Autodesk Inventor part; units mm, degrees
ref_plane "YZ Plane" through (0, 0, 0) normal (1, 0, 0) x (0, 1, 0)
ref_plane "XZ Plane" through (0, 0, 0) normal (0, 1, 0) x (-1, 0, 0)
ref_plane "XY Plane" through (0, 0, 0) normal (0, 0, 1) x (1, 0, 0)
sketch "Sketch2" plane through (0, 0, 0) normal (0, 1, 0) x (-1, 0, 0)
  line L0 (-4, 4) -> (4, 4) construction
  line L1 (4, 4) -> (4, -4) construction
  line L2 (4, -4) -> (-4, -4) construction
  line L3 (-4, -4) -> (-4, 4) construction
  circle A0 centre (0, 0) radius 4
  point P0 (0, 4)
  point P1 (-4, 0)
  dimension "d0" = 8
  dimension "d1" = 8
extrude "Extrusion1" add sketch "Sketch2" along normal blind 3.2
sketch "Sketch10" plane through (0, 0, 0) normal (0, -1, 0) x (1, 0, 0)
  circle A0 centre (0, 0) radius 4
  circle A1 centre (4, 4) radius 2.4 construction
  line L0 (0, 0) -> (4, 4) construction
  circle A2 centre (0, 0) radius 3.2569
  circle A3 centre (0, 0) radius 2.4
  circle A4 centre (0, 0) radius 3.6
  dimension "d92" = 4.8
  dimension "d93" = 4
  dimension "d94" = 4
  dimension "d95" = 4.8
  dimension "d99" = 0.4
extrude "Extrusion6" cut sketch "Sketch10" against normal blind 1.6 contours A3
extrude "Extrusion7" cut sketch "Sketch10" against normal blind 0.4 contours A0
fillet "Fillet1" radius 0.1 1 edges at (4, 3.2, 0)
equation "\"d4\" = 0.333333 * lh"
equation "\"d92\" = kd"
equation "\"d93\" = 0.5 * lu"
equation "\"d94\" = d93"
equation "\"d95\" = kd"
equation "\"d99\" = gw"
equation "\"d96\" = 0.333333 * lh - topthk"
equation "\"d100\" = gh"
properties part number "98138-TransOrange" material "Polycarbonate"
Source: CAD feature listing. Evaluate the final solid. Frame: model axes, mm. A direction names the side the tool comes from. Give positions to 0.01 mm unless a question says otherwise; leave off trailing zeros. Write each loop counter-clockwise with the first axis right and the second up, starting at its lowest first coordinate (ties: lowest second). Pieces come first, ordered by that corner, then holes. Notation, with made-up numbers: M 31.25,-16 L 52.25,-16 A27 cw 52.25,11 Z; hole C -29.5,17 d5. An arc over 180 degrees is marked long. Return JSON: item names as keys, results as strings. Group by question number.
1) Set-up query: faces 4 (the face through (1.29, 0.789, 2.024)), 5 (the face through (0.867, 1.731, 3.905)). Return all of +Z, -Z, +X, -X, +Y, -Y with unobstructed straight access to the full face (end or side cutting, diameter ignored); none if empty.
2) Cut plane B-B, the plane y = 0.8. Output: boundary loops of the cut face in (x, z), plus the area to 3 significant figures.
3) Pull-direction query (Z, two-part tool) for faces 1 (the face through (0, 1.6, 0)), 2 (the face through (0, 3.2, 0)), 3 (the face through (3.434, 0.197, 1.081)); classes: pulls with the +Z half, pulls with the -Z half, needs draft (parallel to the pull), parting line crosses it, or undercut.
4) Pin query (flat end, axial travel): P1, Ø1, axis at y = 0.5, z = -2.5, coming from the +X side; P2, Ø1.5, axis at x = -2.5, y = 2, coming from the +Z side; P3, Ø1, axis at y = 1.5, z = -1, coming from the +X side. Return the tip coordinate at first contact, or that it passes through.
5) Cut plane A-A, the plane z = 0. Output: boundary loops of the cut face in (x, y), plus the area to 3 significant figures.
6) Cut plane D-D, the plane y = 3. Output: boundary loops of the cut face in (x, z), plus the area to 3 significant figures.
7) Material intervals for line 1 along Z through (x, y) = (0, 0.75); line 2 along Z through (x, y) = (0.5, 1.2); line 3 along Y through (x, z) = (-0.5, 0.25), sorted ascending. Write a range as [from, to].
8) Cut plane C-C, the plane x = 0. Output: boundary loops of the cut face in (y, z).
Recorded:
{
 "1": {"face 4": "-Y", "face 5": "+Y, -Y"},
 "2": {"outline": "C 0,0 d8; hole C 0,0 d4.8", "area": "32.2 mm²"},
 "3": {"face 1": "undercut", "face 2": "needs draft", "face 3": "parting line crosses it"},
 "4": {"P1": "stops at x = 3.46", "P2": "stops at z = 3.6", "P3": "stops at x = 3.97"},
 "5": {"outline": "M -4,0.4 L -3.6,0.4 L -3.6,0 L -2.4,0 L -2.4,1.6 L 2.4,1.6 L 2.4,0 L 3.6,0 L 3.6,0.4 L 4,0.4 L 4,3.1 A0.1 ccw 3.9,3.2 L -3.9,3.2 A0.1 ccw -4,3.1 Z", "area": "17.6 mm²"},
 "6": {"outline": "C 0,0 d8", "area": "50.3 mm²"},
 "7": {"line 1": "z = [-4, -2.4], [2.4, 4]", "line 2": "z = [-3.97, -2.35], [2.35, 3.97]", "line 3": "y = [1.6, 3.2]"},
 "8": {"outline": "M 0,-3.6 L 0.4,-3.6 L 0.4,-4 L 3.1,-4 A0.1 ccw 3.2,-3.9 L 3.2,3.9 A0.1 ccw 3.1,4 L 0.4,4 L 0.4,3.6 L 0,3.6 L 0,2.4 L 1.6,2.4 L 1.6,-2.4 L 0,-2.4 Z"}
}
